from build123d import *

# Parameters (mm, degrees)
EXTRUDE_4_DEPTH = 20


with BuildPart() as part:
    # 草图7 → 凸台-拉伸4 (new body)
    with BuildSketch(Plane.XY):
        Polygon((-33.910919067, 18.999592163), (-61.547005384, -28.867513459), (-55.773502692, -38.867513459), (1.462534319, -38.867513459), (55.773502692, -38.867513459), (61.547005384, -28.867513459), (37.633660722, 12.551614473), (5.773502692, 67.735026919), (-5.773502692, 67.735026919), align=None)
        Polygon((-16.951439693, 8.374272109), (0, 37.735026919), (18.097391255, 6.389425782), (32.679491924, -18.867513459), (0.821995205, -18.867513459), (-32.679491924, -18.867513459), align=None, mode=Mode.SUBTRACT)
    extrude(amount=EXTRUDE_4_DEPTH)


solid = part.part
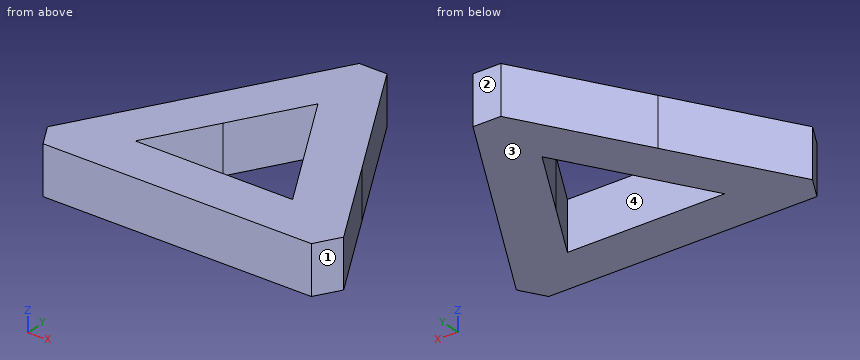
For this review, take the finished solid that the model builds, in its own axes (mm). Face numbers are marked on the shaded views. Round coordinates to 2 decimals unless told otherwise and drop trailing zeros. Order: outer loops, then holes, each group sorted by start corner. A loop starts at its lowest first (then second) coordinate and runs counter-clockwise, first axis right, second up. Notation, with made-up numbers: M -10,-24.75 L -3,-24.75 A19 ccw -3,-17.75 Z; hole C 27.5,-6 d10. An arc over 180 degrees is marked long. Write each question's results on one line, items separated by ' | '. Start each with the question number.
1. Add section A-A (y = -3). State the section outline as (x, z) points, then the cut area to 3 significant figures.
2. Clearance check with flat-ended pins moving along their axes: pin 1 Ø1 at (y, z) = (21, 15.5) entering from -X; pin 2 Ø1 at (y, z) = (-17, 5.5) entering from -X; pin 3 Ø6 at (x, y) = (31.5, -1) entering from -Z; pin 4 Ø10 at (x, z) = (-32, 15) entering from +Y. State where each tip first meets the part, or that it passes through.
3. To check wall thickness, follow L1, parallel to Y at x = -17, z = 15.25; L2, parallel to Y at x = 27, z = 1.25; L3, parallel to X at y = 19, z = 6. State the ranges of each line that lie inside material, in increasing order. Write a range as [from, to].
4. Add section C-C (x = -10). State the section outline as (y, z) points.
5. Add section D-D (y = 42). State the section outline as (x, z) points, then the cut area to 3 significant figures.
6. Add section B-B (z = 2.5). State the section outline as (x, y) points, then the cut area to 3 significant figures.
7. Draft analysis for pull direction Y (two halves, no side actions). For the marked faces 1, 2, 3 and 4, state which applies: pulls with the +Y half, pulls with the -Y half, needs draft (parallel to the pull), parting line crosses it, or undercut.
Output values:
1) outline: M -46.61,0 L -23.52,0 L -23.52,20 L -46.61,20 Z; M 23.52,0 L 46.61,0 L 46.61,20 L 23.52,20 Z | area: 924 mm^2
2) pin 1: x = -33.04 | pin 2: x = -54.98 | pin 3: z = 0 | pin 4: y = 30.97
3) L1: [-38.87, -18.87], [8.29, 48.29] | L2: [-38.87, -18.87], [-9.03, 30.97] | L3: [-33.91, -10.82], [10.82, 33.91]
4) outline: M -38.87,0 L -18.87,0 L -18.87,20 L -38.87,20 Z; M 20.41,0 L 60.41,0 L 60.41,20 L 20.41,20 Z
5) outline: M -20.63,0 L 20.63,0 L 20.63,20 L -20.63,20 Z | area: 825 mm^2
6) outline: M -61.55,-28.87 L -55.77,-38.87 L 55.77,-38.87 L 61.55,-28.87 L 5.77,67.74 L -5.77,67.74 Z; hole M -32.68,-18.87 L 32.68,-18.87 L 0,37.74 Z | area: 5,830 mm^2
7) face 1: pulls with the -Y half | face 2: pulls with the +Y half | face 3: needs draft | face 4: undercut
